Verification items for the finished model (mm, model axes). Coordinates: 2 decimals unless noted, no trailing zeros. Write each loop counter-clockwise with the first axis right and the second up, starting at its lowest first coordinate (ties: lowest second). Pieces come first, ordered by that corner, then holes. Notation, with made-up numbers: M -23.75,53 L 0.25,53 A23 ccw 0.25,81 Z; hole C 41.25,86 d4. An arc over 180 degrees is marked long. One line per item, written item: value.
```python
from build123d import *

# Parameters (mm, degrees)
SKETCH3_W           = 42
SKETCH3_H           = 14
BOSS_EXTRUDE2_DEPTH = 33.5
SKETCH4_R           = 2.6
CUT_EXTRUDE2_DEPTH  = 41.152833026
SKETCH5_R           = 2.6
CUT_EXTRUDE3_DEPTH  = 42.943414263


with BuildPart() as part:
    # Sketch3 → Boss-Extrude2 (new body)
    with BuildSketch(Plane(origin=(0, 0, 0), x_dir=(1, 0, 0), z_dir=(0, 1, 0))):
        Rectangle(SKETCH3_W, SKETCH3_H)
    extrude(amount=BOSS_EXTRUDE2_DEPTH)

    # Sketch4 → Cut-Extrude2 (cut, through all)
    with BuildSketch(Plane(origin=(0, 33.5, 0), x_dir=(1, 0, 0), z_dir=(0, 1, 0))):
        with Locations(Location((-16, 0, 0), (0, 0, 270))):
            Circle(SKETCH4_R)
        with Locations(Location((16, 0, 0), (0, 0, 270))):
            Circle(SKETCH4_R)
    extrude(amount=-CUT_EXTRUDE2_DEPTH, mode=Mode.SUBTRACT)

    # Sketch5 → Cut-Extrude3 (cut, through all)
    with BuildSketch(Plane.XY.offset(7)):
        with Locations((0, 26)):
            Circle(SKETCH5_R)
        with Locations((10, 26)):
            Circle(SKETCH5_R)
        with Locations((-10, 26)):
            Circle(SKETCH5_R)
    extrude(amount=-CUT_EXTRUDE3_DEPTH, mode=Mode.SUBTRACT)


solid = part.part
```
Item 1: Scan lines: line 1 (X direction, y = 18.5, z = 0); line 2 (Y direction, x = -10, z = 0); line 3 (X direction, y = 29.5, z = -2). Record each from-to range of solid material in increasing order.
The answers:
line 1: x = -21 to -18.6, -13.4 to 13.4, 18.6 to 21
line 2: y = 0 to 23.4, 28.6 to 33.5
line 3: x = -21 to -17.66, -14.34 to 14.34, 17.66 to 21
Item 2: Cross-section at B-B, the plane x = 16. Enter the section's corners in (y, z), and give its area (3 significant figures).
The answers:
outline: M 0,-7 L 33.5,-7 L 33.5,-2.6 L 0,-2.6 Z; M 0,2.6 L 33.5,2.6 L 33.5,7 L 0,7 Z
area: 295 mm²
Item 3: Cross-section at D-D, the plane z = -3.75. Enter the section's corners in (x, y).
The answers:
outline: M -21,0 L 21,0 L 21,33.5 L -21,33.5 Z; hole C -10,26 d5.2; hole C 0,26 d5.2; hole C 10,26 d5.2
Item 4: Cross-section at C-C, the plane y = 26. Enter the section's corners in (x, z).
The answers:
outline: M -21,-7 L -12.6,-7 L -12.6,7 L -21,7 Z; M -7.4,-7 L -2.6,-7 L -2.6,7 L -7.4,7 Z; M 2.6,-7 L 7.4,-7 L 7.4,7 L 2.6,7 Z; M 12.6,-7 L 21,-7 L 21,7 L 12.6,7 Z; hole C -16,0 d5.2; hole C 16,0 d5.2
Item 5: Draft check along X on faces 1 (the face through (0, 17, -7)), 2 (the face through (21, 17, 0)), 3 (the face through (13.693, 16.984, 1.2)). Enter one of: released by +X, released by -X, zero draft, split by the parting line, or undercut.
The answers:
face 1: zero draft
face 2: released by +X
face 3: undercut
Item 6: Cross-section at A-A, the plane z = 0. Enter the section's corners in (x, y).
The answers:
outline: M -21,0 L -18.6,0 L -18.6,33.5 L -21,33.5 Z; M -13.4,0 L 13.4,0 L 13.4,33.5 L -13.4,33.5 Z; M 18.6,0 L 21,0 L 21,33.5 L 18.6,33.5 Z; hole C -10,26 d5.2; hole C 0,26 d5.2; hole C 10,26 d5.2
